Could you check a few things on this model? Use its own coordinates, in mm. Round coordinates to 2 decimals unless told otherwise and drop trailing zeros. Write each loop counter-clockwise with the first axis right and the second up, starting at its lowest first coordinate (ties: lowest second). Pieces come first, ordered by that corner, then holes. Notation, with made-up numbers: (19.25, 25.25) -> (48.25, 25.25) arc R16 cw to (48.25, 46.25) -> close; hole circle Ø6 at (-22, 86.5). An arc over 180 degrees is marked (long way). Answer in a Markdown table with one row per item. Add a question column.
```python
from build123d import *

# Parameters (mm, degrees)
F0_W     = 19.1008
F0_H     = 34.925
F0_W_2   = 72.136
F0_H_2   = 19.1008
F0_W_3   = 96.012
F0_H_3   = 279.4
F0_W_4   = 19.431
F0_H_4   = 62.737998
F0_W_5   = 19.3548
F0_H_5   = 62.738
F0_H_6   = 62.992
F0_R     = 26.025224
F1_DEPTH = 25.4


with BuildPart() as f1:
    # F0 (on Front) → F1 (new body)
    with BuildSketch(Plane.XZ):
        Polygon((12.727918, 557.499766), (-467.555925, 166.415552), (-368.272082, 42.7843), (-368.272082, -618.276235), (-368.272082, -1136.548519), (393.727918, -1136.548519), (393.727918, -618.276235), (393.727918, 42.7843), (493.011761, 166.415552), align=None)
        with Locations((-270.224877, -925.450377)):
            Rectangle(F0_W, F0_H, mode=Mode.SUBTRACT)
        with Locations((-194.402747, -983.356682)):
            Rectangle(F0_W_2, F0_H_2, mode=Mode.SUBTRACT)
        with Locations((-1.08871, -930.430109)):
            Rectangle(F0_W_3, F0_H_3, mode=Mode.SUBTRACT)
        with Locations((-194.402747, -872.307882)):
            Rectangle(F0_W_2, F0_H_2, mode=Mode.SUBTRACT)
        with Locations((-203.619584, -625.265823)):
            Rectangle(F0_W_4, F0_H_4, mode=Mode.SUBTRACT)
        with Locations((-203.6826, -486.327824)):
            Rectangle(F0_W_5, F0_H_5, mode=Mode.SUBTRACT)
        with Locations((-203.828264, -347.262824)):
            Rectangle(F0_W, F0_H_6, mode=Mode.SUBTRACT)
        with Locations((203.454484, -625.646824)):
            Rectangle(F0_W, F0_H_6, mode=Mode.SUBTRACT)
        with Locations((203.4794, -486.454824)):
            Rectangle(F0_W, F0_H_6, mode=Mode.SUBTRACT)
        with Locations((203.828264, -347.262824)):
            Rectangle(F0_W, F0_H_6, mode=Mode.SUBTRACT)
        with Locations((-203.807441, -208.070824)):
            Rectangle(F0_W, F0_H_6, mode=Mode.SUBTRACT)
        with Locations((0, 187.761217)):
            Circle(F0_R, mode=Mode.SUBTRACT)
        with Locations((203.642379, -208.070824)):
            Rectangle(F0_W_4, F0_H_6, mode=Mode.SUBTRACT)
    extrude(amount=F1_DEPTH)


solid = f1.part
```
(1) Suppose I cut it at B-B, the plane x = -299. Please give me the cut outline in (y, z), then the cut area to 3 significant figures.
(2) Suppose I cut it at C-C, the plane y = -21.5. State how many separate pieces and enclosed holes the cut face has, then the cut area to 3 significant figures.
(3) For P1, Ø1, axis at y = -6.5, z = 89.5, coming from the -X side; P2, Ø6, axis at y = -20.5, z = -296, coming from the -X side; P3, Ø2, axis at x = -177, y = -14.5, coming from the +Z side, each with a flat end and sliding along its axis, tell me the tip position at first contact or that it passes through.
(4) If we mould it in two halves opening along Z, with no side actions, what happens to faces 1 (the face through (6, 0, -278)), 2 (the face through (24.823, -12.522, 195.578)), 3 (the face through (-224.052, -12.522, 364.695))? For each: pulls with the +Z half, pulls with the -Z half, needs draft (parallel to the pull), parting line crosses it, or undercut.
(5) I need wall thicknesses on L1, parallel to X at y = -5.25, z = -195; L2, parallel to Z at x = 0, y = -13; L3, parallel to X at y = -4, z = -897.5. Which ranges of each line are inside material? Lowest first, please.
(6) Suppose I cut it at A-A, the plane z = -475. Please give me the cut outline in (x, y), then the cut area to 3 significant figures.
(7) Suppose I cut it at D-D, the plane x = 344. Please give me the cut outline in (y, z), then the cut area to 3 significant figures.
Response:
| question | item | result |
|---|---|---|
| 1 | outline | (-25.4, -1136.55) -> (0, -1136.55) -> (0, 303.67) -> (-25.4, 303.67) -> close |
| 1 | area | 36,600 mm² |
| 2 | separate pieces | 1 |
| 2 | enclosed holes | 13 |
| 2 | area | 1,150,000 mm² |
| 3 | P1 | x = -406.19 |
| 3 | P2 | x = -368.27 |
| 3 | P3 | z = 403.82 |
| 4 | face 1 | needs draft |
| 4 | face 2 | undercut |
| 4 | face 3 | pulls with the +Z half |
| 5 | L1 | -368.27 to -213.36, -194.26 to 193.93, 213.36 to 393.73 |
| 5 | L2 | -1136.55 to -1070.13, -790.73 to 161.74, 213.79 to 547.14 |
| 5 | L3 | -368.27 to -49.09, 46.92 to 393.73 |
| 6 | outline | (-368.27, -25.4) -> (-213.36, -25.4) -> (-213.36, 0) -> (-368.27, 0) -> close; (-194.01, -25.4) -> (193.93, -25.4) -> (193.93, 0) -> (-194.01, 0) -> close; (213.03, -25.4) -> (393.73, -25.4) -> (393.73, 0) -> (213.03, 0) -> close |
| 6 | area | 18,400 mm² |
| 7 | outline | (-25.4, -1136.55) -> (0, -1136.55) -> (0, 287.75) -> (-25.4, 287.75) -> close |
| 7 | area | 36,200 mm² |
